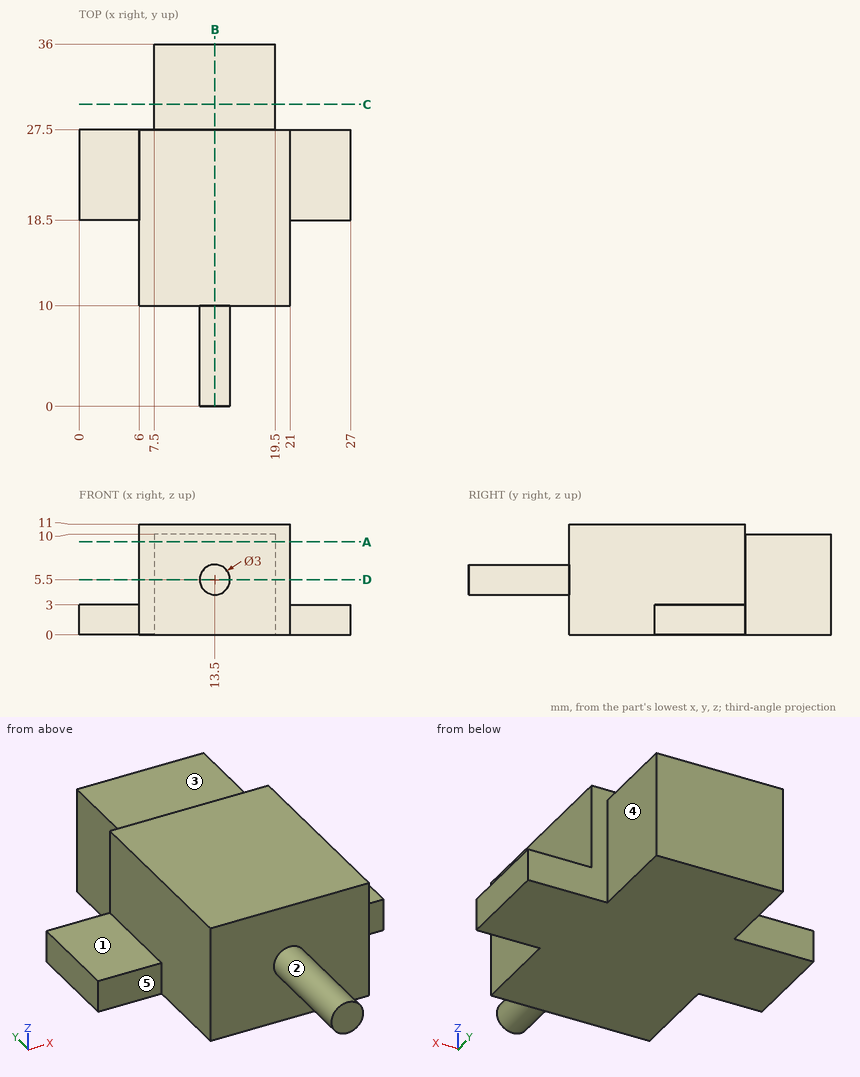
Geometry check sheet. Reference: drawing and pictorial views, mm from the part's lowest x, y, z. A direction names the side the tool comes from. Coordinates: 2 decimals unless noted, no trailing zeros. Order: outer loops, then holes, each group sorted by start corner. A loop starts at its lowest first (then second) coordinate and runs counter-clockwise, first axis right, second up.
1. Sectioned sample at A-A, the plane z = 9.25. Record the cut outline in (x, y).
Results found:
outline: (6, 10) - (21, 10) - (21, 27.5) - (19.5, 27.5) - (19.5, 36) - (7.5, 36) - (7.5, 27.5) - (6, 27.5) - close
2. Go/stop test with flat-tipped pins: pin 1 Ø2.5 at (y, z) = (33.5, 2.5) entering from -X; pin 2 Ø4 at (x, y) = (11.5, 34) entering from +Z; pin 3 Ø3 at (x, y) = (25, 21) entering from +Z. Record where each tip stops, or that it passes through.
Results found:
pin 1: stops at x = 7.5
pin 2: stops at z = 10
pin 3: stops at z = 3
3. Sectioned sample at D-D, the plane z = 5.5. Record the cut outline in (x, y), and give its area (4 significant figures).
Results found:
outline: (6, 10) - (12, 10) - (12, 0) - (15, 0) - (15, 10) - (21, 10) - (21, 27.5) - (19.5, 27.5) - (19.5, 36) - (7.5, 36) - (7.5, 27.5) - (6, 27.5) - close
area: 394.5 mm2
4. Scan lines: line 1 (X direction, y = 11.5, z = 5); line 2 (Y direction, x = 20, z = 7.5); line 3 (Z direction, x = 25.75, y = 25). Record each from-to range of solid material in increasing order.
Results found:
line 1: x = 6 to 21
line 2: y = 10 to 27.5
line 3: z = 0 to 3
5. Sectioned sample at C-C, the plane y = 30. Record the cut outline in (x, z), and give its area (3 significant figures).
Results found:
outline: (7.5, 0) - (19.5, 0) - (19.5, 10) - (7.5, 10) - close
area: 120 mm2
6. Set-up check for the marked faces 1, 2, 3, 4 and 5: record each of +Z, -Z, +X, -X, +Y, -Y from which the full face is reachable in a straight line by a thin tool's end or side.
Results found:
face 1: +Z, -X, +Y, -Y
face 2: -Y
face 3: +Z, +X, -X, +Y
face 4: +Z, -Z, +X, +Y
face 5: +Z, -Z, -X, -Y
7. Sectioned sample at B-B, the plane x = 13.5. Record the cut outline in (y, z).
Results found:
outline: (0, 4) - (10, 4) - (10, 0) - (36, 0) - (36, 10) - (27.5, 10) - (27.5, 11) - (10, 11) - (10, 7) - (0, 7) - close
